Autodesk Inventor part; units mm, degrees
ref_plane "YZ Plane" through (0, 0, 0) normal (1, 0, 0) x (0, 1, 0)
ref_plane "XZ Plane" through (0, 0, 0) normal (0, 1, 0) x (-1, 0, 0)
ref_plane "XY Plane" through (0, 0, 0) normal (0, 0, 1) x (1, 0, 0)
sketch "main" plane through (0, 0, 0) normal (0, 0, 1) x (1, 0, 0)
  circle A0 centre (-16.6212, -19.5437) radius 2.1844
  arc A1 (-20.9032, -24.2328) -> (-16.6212, -25.8937) centre (-16.6212, -19.5437) ccw
  circle A2 centre (-22.9712, 9.4504) radius 2.0955
  arc A3 (-13.0318, 36.2391) -> (-20.24, 36.2816) centre (-16.6667, 31.0324) ccw
  line L0 (-20.9032, -24.2328) -> (-52.6534, 4.7613)
  circle A4 centre (-35.6713, 9.4504) radius 2.0955
  circle A5 centre (-48.3714, 9.4504) radius 2.0955
  arc A6 (-51.9447, 14.6996) -> (-52.6534, 4.7613) centre (-48.3714, 9.4504) ccw
  line L1 (-20.24, 36.2816) -> (-51.9447, 14.6996)
  circle A7 centre (46.8788, -19.5437) radius 2.1844
  arc A8 (46.8788, -25.8937) -> (53.2288, -19.5437) centre (46.8788, -19.5437) ccw
  line L2 (47.7986, -6.2278) -> (-13.0318, 36.2391)
  line L3 (46.8788, -25.8937) -> (-16.6212, -25.8937)
  arc A9 (53.2288, -16.6412) -> (47.7986, -6.2278) centre (40.5288, -16.6412) ccw
  line L4 (53.2288, -19.5437) -> (53.2288, -16.6412)
  point P0 (0.102, -2.5446)
  point P1 (53.2288, -10.0187)
  dimension "d0" = 12.7
  dimension "d1" = 9.525
  dimension "d2" = 12.7
  dimension "d3" = 12.7
  dimension "d4" = 6.35
  dimension "d5" = 4.191
  dimension "d6" = 4.191
  dimension "d7" = 4.191
sketch "Sketch1" plane through (0, 0, 0) normal (0, 0, 1) x (1, 0, 0)
  circle A0 centre (63.5, 0) radius 2.1844
  arc A1 (67.782, 4.689) -> (63.5, 6.35) centre (63.5, 0) ccw
  circle A2 centre (69.85, -28.9941) radius 2.0955
  arc A3 (59.9106, -55.7828) -> (67.1187, -55.8253) centre (63.5455, -50.5761) ccw
  line L0 (67.782, 4.689) -> (99.5322, -24.3051)
  circle A4 centre (82.55, -28.9941) radius 2.0955
  circle A5 centre (95.2502, -28.9941) radius 2.0955
  arc A6 (98.8235, -34.2433) -> (99.5322, -24.3051) centre (95.2502, -28.9941) ccw
  line L1 (67.1187, -55.8253) -> (98.8235, -34.2433)
  circle A7 centre (0, 0) radius 2.1844
  arc A8 (0, 6.35) -> (-6.35, 0) centre (0, 0) ccw
  line L2 (-0.9198, -13.3159) -> (59.9106, -55.7828)
  line L3 (0, 6.35) -> (63.5, 6.35)
  arc A9 (-6.35, -2.9025) -> (-0.9198, -13.3159) centre (6.35, -2.9025) ccw
  line L4 (-6.35, 0) -> (-6.35, -2.9025)
  point P0 (0, 0)
extrude "Extrusion1" add sketch "Sketch1" along normal blind 1.5875
properties part number "sled" material "Acetal Resin, White"
Geometry: final body of the model. Coordinates: model frame, mm. Round coordinates to 2 decimals unless told otherwise and drop trailing zeros. Loops run counter-clockwise (first coordinate to the right, second up) from the corner with the lowest first, then second, coordinate; pieces in that order, holes last.
Q1. Pull-direction query (Y, two-part tool) for faces 1 (the cylindrical face through (101.59, -29.37, 0.78)), 2 (the cylindrical face through (80.457, -29.086, 0.783)), 3 (the flat face through (83.435, -9.605, 0.783)); classes: released by +Y, released by -Y, zero draft, split by the parting line, or undercut.
Q2. Section C-C on x = 69.85. Return loops of the section in (y, z), plus the area to 3 significant figures.
Q3. Material intervals for L1, parallel to Y at x = 63.5, z = 0.85; L2, parallel to Y at x = 82.55, z = 1.15; L3, parallel to X at y = -34.5, z = 0.1, sorted ascending.
Q4. Pin query (flat end, axial travel): P1, Ø2.5, axis at x = 63.5, y = 0, coming from the -Z side. Return the tip coordinate at first contact, or that it passes through.
Q5. Section D-D on y = -21. Return loops of the section in (x, z), plus the area to 3 significant figures.
Q6. Section A-A on x = 82.55. Return loops of the section in (y, z).
Q7. Section B-B on z = 0.3. Return loops of the section in (x, y), plus the area to 3 significant figures.
Evaluation:
1. face 1: split by the parting line
1. face 2: undercut
1. face 3: released by +Y
2. outline: (-53.97, 0) - (-31.09, 0) - (-31.09, 1.59) - (-53.97, 1.59) - close; (-26.9, 0) - (2.8, 0) - (2.8, 1.59) - (-26.9, 1.59) - close
2. area: 83.5 mm2
3. L1: y = -56.93 to -2.18, 2.18 to 6.35
3. L2: y = -45.32 to -31.09, -26.9 to -8.8
3. L3: x = 29.42 to 98.45
4. P1: passes through
5. outline: (10.09, 0) - (95.91, 0) - (95.91, 1.59) - (10.09, 1.59) - close
5. area: 136 mm2
6. outline: (-45.32, 0) - (-31.09, 0) - (-31.09, 1.59) - (-45.32, 1.59) - close; (-26.9, 0) - (-8.8, 0) - (-8.8, 1.59) - (-26.9, 1.59) - close
7. outline: (-6.35, -2.9) arc R12.7 ccw to (-0.92, -13.32) - (59.91, -55.78) arc R6.35 ccw to (67.12, -55.83) - (98.82, -34.24) arc R6.35 ccw to (99.53, -24.31) - (67.78, 4.69) arc R6.35 ccw to (63.5, 6.35) - (0, 6.35) arc R6.35 ccw to (-6.35, 0) - close; hole circle Ø4.37 at (0, 0); hole circle Ø4.37 at (63.5, 0); hole circle Ø4.19 at (69.85, -28.99); hole circle Ø4.19 at (82.55, -28.99); hole circle Ø4.19 at (95.25, -28.99)
7. area: 4,110 mm2
